Here's how the part is built. I have some questions about the finished solid (model axes, mm). Face numbers are marked on the shaded views. A direction names the side the tool comes from. Coordinates: 2 decimals unless noted, no trailing zeros. Write each loop counter-clockwise with the first axis right and the second up, starting at its lowest first coordinate (ties: lowest second). Pieces come first, ordered by that corner, then holes.
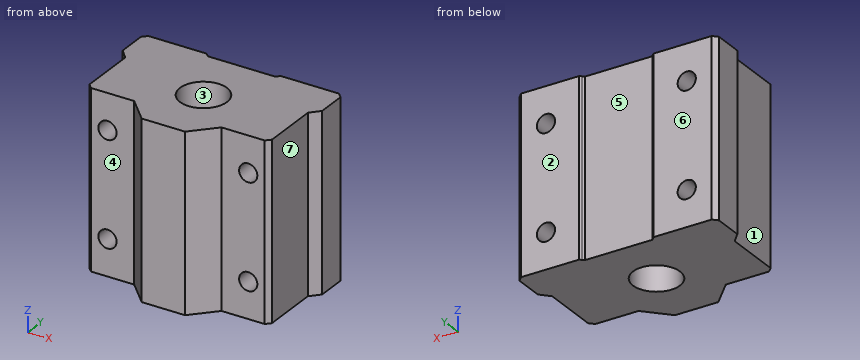
```python
from build123d import *

# Parameters (mm, degrees)
SKETCH1_R           = 4
BOSS_EXTRUDE1_DEPTH = 30
SKETCH2_R           = 1.5494
CUT_EXTRUDE1_DEPTH  = 49.630200751
SKETCH3_W           = 12.065
SKETCH3_H           = 30
CUT_EXTRUDE2_DEPTH  = 0.5842
CHAMFER1_SIZE       = 0.2921
CUT_EXTRUDE3_DEPTH  = 51.171756524
CHAMFER2_SIZE       = 0.762


with BuildPart() as part:
    # Sketch1 → Boss-Extrude1 (new body)
    with BuildSketch(Plane.XY):
        Polygon((0, 0), (33.9598, 0), (33.9598, -17.653), (24.4094, -17.653), (20.6629, -21.5392), (13.2969, -21.5392), (9.5504, -17.653), (0, -17.653), align=None)
        with Locations((16.9799, -10.7696)):
            Circle(SKETCH1_R, mode=Mode.SUBTRACT)
    extrude(amount=BOSS_EXTRUDE1_DEPTH)

    # Sketch2 → Cut-Extrude1 (cut, through all)
    with BuildSketch(Plane(origin=(0, -17.653, 0), x_dir=(-1, 0, 0), z_dir=(0, -1, 0))):
        with Locations(Location((-5.0038, -23.8773, 0), (0, 0, 90))):
            Circle(SKETCH2_R)
        with Locations(Location((-5.0038, -6.1227, 0), (0, 0, 90))):
            Circle(SKETCH2_R)
        with Locations(Location((-28.956, -6.1227, 0), (0, 0, 90))):
            Circle(SKETCH2_R)
        with Locations(Location((-28.956, -23.8773, 0), (0, 0, 90))):
            Circle(SKETCH2_R)
    extrude(amount=-CUT_EXTRUDE1_DEPTH, mode=Mode.SUBTRACT)

    # Sketch3 → Cut-Extrude2 (cut)
    with BuildSketch(Plane(origin=(0, 0, 0), x_dir=(1, 0, 0), z_dir=(0, 1, 0))):
        with Locations((16.9799, -15)):
            Rectangle(SKETCH3_W, SKETCH3_H)
    extrude(amount=-CUT_EXTRUDE2_DEPTH, mode=Mode.SUBTRACT)

    # Chamfer1
    chamfer1_edges = [part.edges().sort_by_distance(p)[0] for p in [
        (23.0124, -0.5842, 15),
        (10.9474, -0.5842, 15),
    ]]
    chamfer(chamfer1_edges, length=CHAMFER1_SIZE)
    chamfer1_2_edges = [part.edges().sort_by_distance(p)[0] for p in [
        (23.0124, 0, 15),
        (10.9474, 0, 15),
    ]]
    chamfer(chamfer1_2_edges, length=CHAMFER1_SIZE - 0.0001)  # a hair under: the kernel refuses the full size

    # Sketch4 → Cut-Extrude3 (cut, through all)
    with BuildSketch(Plane.XY.offset(30)):
        Polygon((1.4478, -17.653), (1.4478, -7.2644), (0, -5.6896), (0, -17.653), align=None)
    cut_extrude3 = extrude(amount=-CUT_EXTRUDE3_DEPTH, mode=Mode.SUBTRACT)

    # Mirror1: Cut-Extrude3 across plane
    add(cut_extrude3.mirror(Plane.ZY.offset(-16.9799)), mode=Mode.SUBTRACT)

    # Chamfer2
    chamfer2_edges = [part.edges().sort_by_distance(p)[0] for p in [
        (32.512, -17.653, 15),
        (0, 0, 15),
        (33.9598, 0, 15),
        (1.4478, -17.653, 15),
    ]]
    chamfer(chamfer2_edges, length=CHAMFER2_SIZE)


solid = part.part
```
1) Imagine slicing it at C-C on x = 15.5. Please give me the cut outline in (y, z).
Values follow:
outline: (-21.54, 0) - (-14.49, 0) - (-14.49, 30) - (-21.54, 30) - close; (-7.05, 0) - (-0.58, 0) - (-0.58, 30) - (-7.05, 30) - close
2) Will these pins go through, and if not, where does the flat tip stop? pin 1 (8 mm diameter, centred on y = -11.5, z = 22.5, fed in from -X); pin 2 (1 mm diameter, centred on x = 27.5, z = 25, fed in from -Y); pin 3 (3 mm diameter, centred on y = -11.5, z = 22, fed in from +X).
Values follow:
pin 1: stops at x = 1.45
pin 2: stops at y = -17.65
pin 3: stops at x = 32.51
3) Imagine slicing it at A-A on y = -11.5. Please give me the cut outline in (x, z).
Values follow:
outline: (1.45, 0) - (13.05, 0) - (13.05, 30) - (1.45, 30) - close; (20.91, 0) - (32.51, 0) - (32.51, 30) - (20.91, 30) - close; hole circle Ø3.1 at (5, 6.12); hole circle Ø3.1 at (5, 23.88); hole circle Ø3.1 at (28.96, 6.12); hole circle Ø3.1 at (28.96, 23.88)
4) I need wall thicknesses on probe 1 along Z at (x, y) = (29, -10.25); probe 2 along X at (y, z) = (-9.5, 6.5); probe 3 along Z at (x, y) = (30, -2.5). Which ranges of each line are inside material? Lowest first, please.
Values follow:
probe 1: z = 0 to 4.57, 7.67 to 22.33, 25.43 to 30
probe 2: x = 1.45 to 3.5, 6.51 to 13.19, 20.77 to 27.45, 30.46 to 32.51
probe 3: z = 0 to 4.98, 7.27 to 22.73, 25.02 to 30
5) On a 3-axis mill with a long thin cutter (end or side, diameter ignored), from which of +Z, -Z, +X, -X, +Y, -Y can I reach the whole of each face in a straight line? I mean the marked faces 4, 5, 6 and 7. Say none if no direction works.
Values follow:
face 4: +Z, -Z, -X, -Y
face 5: +Z, -Z, +Y
face 6: +Z, -Z, +X, -X, +Y
face 7: +Z, -Z, +X, -Y
6) We'd pull the mould along X, two halves only. Please class the marked faces 1, 2 and 3: pulls with the +X half, pulls with the -X half, needs draft (parallel to the pull), parting line crosses it, or undercut.
Values follow:
face 1: pulls with the -X half
face 2: needs draft
face 3: undercut
7) Imagine slicing it at B-B on z = 25. Count the separate pieces of the cut face and the enclosed holes in it, then the cut area to 3 significant figures.
Values follow:
separate pieces: 3
enclosed holes: 1
area: 476 mm2
8) Imagine slicing it at D-D on y = -5.25. Please give me the cut outline in (x, z), then the cut area to 3 significant figures.
Values follow:
outline: (0, 0) - (33.96, 0) - (33.96, 30) - (0, 30) - close; hole circle Ø3.1 at (5, 6.12); hole circle Ø3.1 at (5, 23.88); hole circle Ø3.1 at (28.96, 6.12); hole circle Ø3.1 at (28.96, 23.88)
area: 989 mm2
